The model under review builds one solid part; all positions refer to its coordinate system, in mm. A direction names the side the tool comes from. Round coordinates to 2 decimals unless told otherwise and drop trailing zeros. Write each loop counter-clockwise with the first axis right and the second up, starting at its lowest first coordinate (ties: lowest second). Pieces come first, ordered by that corner, then holes.
Item 1: Add section A-A (x = 0). Give the boundary of the cut face in (y, z), plus the area to 3 significant figures.
Item 2: Clearance check with flat-ended pins moving along their axes: pin 1 Ø1.5 at (y, z) = (22, 0) entering from -X; pin 2 Ø0.9 at (y, z) = (29.5, 0) entering from -X; pin 3 Ø1.8 at (x, y) = (16.48, 16.5) entering from -Z; pin 4 Ø0.9 at (y, z) = (-18, -0.5) entering from +X. State where each tip first meets the part, or that it passes through.
Item 3: Draft analysis for pull direction Y (two halves, no side actions). For faces 1 (the face through (-15, 31.5, 0)), 2 (the face through (26, 25, 0)), 3 (the face through (0, 0, 1.5)), state which applies: +Y half, -Y half, draft (parallel to the pull), parting line (faces both ways), or undercut.
Item 4: Add section B-B (y = 16.5). Give the boundary of the cut face in (x, z), plus the area to 3 significant figures.
Item 5: Add section C-C (z = 0.4). State how many separate pieces and enclosed holes the cut face has, plus the area to 3 significant figures.
Item 6: Machinability: for faces 4 (the face through (-25.021, -20, 0)), 5 (the face through (26, -25, 0)), 6 (the face through (-8.75, -30, 0)), 7 (the face through (-20, 30, 0)), 8 (the face through (-19, -31.5, 0)), which of the approach directions +Z, -Z, +X, -X, +Y, -Y give a long, thin tool a straight path to every point of the face, cutting with its end or side? Answer none if there is none.
Item 7: To check wall thickness, follow L1, parallel to Y at x = -11.43, z = -0.5; L2, parallel to X at y = -13, z = 1.3; L3, parallel to X at y = -21, z = -0.25. State the ranges of each line that lie inside material, in increasing order.
Autodesk Inventor part; units mm, degrees
ref_plane "YZ Plane" through (0, 0, 0) normal (1, 0, 0) x (0, 1, 0)
ref_plane "XZ Plane" through (0, 0, 0) normal (0, 1, 0) x (-1, 0, 0)
ref_plane "XY Plane" through (0, 0, 0) normal (0, 0, 1) x (1, 0, 0)
sketch "Sketch1" plane through (0, 0, 0) normal (0, 0, 1) x (1, 0, 0)
  circle A0 centre (16.4791, 16.5) radius 1.5
  circle A1 centre (16.4791, -2.25) radius 1.5
  line L0 (8.75, -28.5) -> (8.75, -31.5)
  line L1 (25.0209, -31.5) -> (8.75, -31.5)
  line L2 (-8.75, -28.5) -> (8.75, -28.5)
  circle A2 centre (11.43, -16.1838) radius 8.115
  circle A3 centre (19.05, -8.9448) radius 1.5875
  circle A4 centre (-19.05, -23.4228) radius 1.5875
  circle A5 centre (0, -9.5798) radius 2.5
  circle A6 centre (-11.43, -16.1838) radius 8.115
  line L3 (0, 8) -> (0, 18) construction
  line L4 (0, 18) -> (8.75, 18) construction
  line L5 (5, 31.5) -> (-5, 31.5)
  line L6 (-5, 28.5) -> (5, 31.5) construction
  line L7 (5, 28.5) -> (-5, 31.5) construction
  line L8 (-5, 28.5) -> (5, 28.5) construction
  line L9 (20, 31.5) -> (10, 31.5)
  line L10 (-10, 31.5) -> (-20, 31.5)
  line L11 (5, 31.5) -> (-5, 31.5)
  line L12 (-10, 28.5) -> (-10, 31.5)
  line L13 (-20, 28.5) -> (-20, 31.5)
  line L14 (10, 28.5) -> (10, 31.5)
  line L15 (20, 31.5) -> (20, 28.5)
  line L16 (-10, 28.5) -> (-5, 28.5)
  line L17 (5, 28.5) -> (10, 28.5)
  line L18 (-28.0209, -5) -> (-28.0209, -15)
  line L19 (-28.0209, -15) -> (-25.0209, -15)
  line L20 (-25.0209, -25) -> (-28.0209, -25)
  line L21 (-28.0209, -25) -> (-28.0209, -31.5)
  line L22 (-28.0209, -5) -> (-25.0209, -5)
  line L23 (-28.0209, 5) -> (-25.0209, 5)
  line L24 (-28.0209, 5) -> (-28.0209, 15)
  line L25 (-28.0209, 15) -> (-25.0209, 15)
  line L26 (-25.0209, 25) -> (-28.0209, 25)
  line L27 (-28.0209, 25) -> (-28.0209, 28.5)
  line L28 (-28.0209, 28.5) -> (-20, 28.5)
  line L29 (-25.0209, 15) -> (-25.0209, 25)
  line L30 (-25.0209, -25) -> (-25.0209, -15)
  line L31 (-25.0209, -5) -> (-25.0209, 5)
  line L32 (28.0209, -5) -> (28.0209, -15)
  line L33 (28.0209, -15) -> (25.0209, -15)
  line L34 (25.0209, -25) -> (28.0209, -25)
  line L35 (28.0209, -25) -> (28.0209, -31.5)
  line L36 (28.0209, -31.5) -> (25.0209, -31.5)
  line L37 (28.0209, -5) -> (25.0209, -5)
  line L38 (28.0209, 5) -> (25.0209, 5)
  line L39 (28.0209, 5) -> (28.0209, 15)
  line L40 (28.0209, 15) -> (25.0209, 15)
  line L41 (25.0209, 25) -> (28.0209, 25)
  line L42 (28.0209, 25) -> (28.0209, 28.5)
  line L43 (28.0209, 28.5) -> (20, 28.5)
  line L44 (25.0209, 15) -> (25.0209, 25)
  line L45 (25.0209, -25) -> (25.0209, -15)
  line L46 (25.0209, -5) -> (25.0209, 5)
  line L47 (-8.75, -31.5) -> (-8.75, -28.5)
  line L48 (-28.0209, -31.5) -> (-8.75, -31.5)
  line L49 (-5, 28.5) -> (-5, 31.5)
  line L50 (5, 28.5) -> (5, 31.5)
  point P0 (0, 0)
  point P1 (0, 30)
  dimension "d2" = 3
  dimension "d5" = 15
  dimension "d8" = 15
  dimension "d12" = 5
  dimension "d13" = 10
  dimension "d16" = 3
  dimension "d17" = 3
extrude "Extrusion2" add sketch "Sketch1" along normal mid plane 3
properties part number "srfdiagkiri"
Numbers:
1. outline: (-28.5, -1.5) - (-12.08, -1.5) - (-12.08, 1.5) - (-28.5, 1.5) - close; (-7.08, -1.5) - (31.5, -1.5) - (31.5, 1.5) - (-7.08, 1.5) - close
1. area: 165 mm2
2. pin 1: stops at x = -25.02
2. pin 2: stops at x = -20
2. pin 3: passes through
2. pin 4: stops at x = 25.02
3. face 1: +Y half
3. face 2: undercut
3. face 3: draft
4. outline: (-25.02, -1.5) - (14.98, -1.5) - (14.98, 1.5) - (-25.02, 1.5) - close; (17.98, -1.5) - (25.02, -1.5) - (25.02, 1.5) - (17.98, 1.5) - close
4. area: 141 mm2
5. separate pieces: 1
5. enclosed holes: 7
5. area: 2,760 mm2
6. face 4: +Z, -Z, -X
6. face 5: +Z, -Z, +X
6. face 6: +Z, -Z, -Y
6. face 7: +Z, -Z, -X, +Y
6. face 8: +Z, -Z, +X, -X, -Y
7. L1: y = -31.5 to -24.3, -8.07 to 31.5
7. L2: x = -28.02 to -18.89, -3.97 to 3.97, 18.89 to 28.02
7. L3: x = -25.02 to -17.96, -4.9 to 4.9, 17.96 to 25.02
